Part model, mm, in its own coordinate system. Face numbers are marked on the shaded views. Round coordinates to 2 decimals unless told otherwise and drop trailing zeros. Write each loop counter-clockwise with the first axis right and the second up, starting at its lowest first coordinate (ties: lowest second). Pieces come first, ordered by that corner, then holes. Notation, with made-up numbers: (46, 47.5) -> (103, 47.5) arc R17 ccw to (103, 69.5) -> close; hole circle Ø4 at (71.5, 13). An arc over 180 degrees is marked (long way). Use CSV: the item, a comma, the result in double quotes. Start each with the question number.
(1) Two-plate mould, pull along Z, no slides. Class the marked faces 1, 2, 3 and 4: released by +Z, released by -Z, zero draft, split by the parting line, or undercut.
(2) Saw through at C-C (z = 0.5). Give the cut face in (x, y).
(3) Saw through at A-A (y = 0.9). Give the cut face in (x, z), plus the area to 3 significant figures.
(4) Drop a flat-ended pin along its axis: pin 1 (1.5 mm diameter, centred on x = 0.5, z = 0.5, fed in from -Y). Give the stop position or say it passes through.
(5) Probe line 1 (Z direction, x = -0.75, y = 1.75); line 2 (X direction, y = 1.8, z = 2); line 3 (Y direction, x = -1, z = 0). List the from-to ranges inside material, lowest first. Write a range as [from, to].
(6) Saw through at B-B (x = 1). Give the cut face in (y, z), plus the area to 3 significant figures.
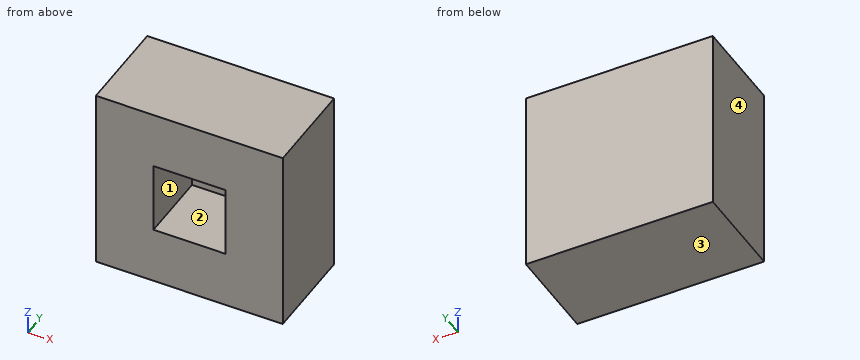
```python
from build123d import *

# Parameters (mm, degrees)
SKETCH1_W           = 7.8
SKETCH1_H           = 7.8
BOSS_EXTRUDE1_DEPTH = 3
SKETCH3_W           = 7.8
SKETCH3_H           = 7.8
BOSS_EXTRUDE2_DEPTH = 1
CUT_EXTRUDE1_DEPTH  = 3


with BuildPart() as part:
    # Sketch1 → Boss-Extrude1 (new body)
    with BuildSketch(Plane(origin=(0, 0, 0), x_dir=(1, 0, 0), z_dir=(0, 1, 0))):
        with Locations((0.315714286, -0.742857143)):
            Rectangle(SKETCH1_W, SKETCH1_H)
    extrude(amount=BOSS_EXTRUDE1_DEPTH)

    # Sketch3 → Boss-Extrude2 (add)
    with BuildSketch(Plane(origin=(0, 3, 0), x_dir=(1, 0, 0), z_dir=(0, 1, 0))):
        with Locations((0.315714286, -0.742857143)):
            Rectangle(SKETCH3_W, SKETCH3_H)
    extrude(amount=BOSS_EXTRUDE2_DEPTH)

    # Sketch4 → Cut-Extrude1 (cut)
    with BuildSketch(Plane.XZ):
        Polygon((0.319353372, 2.24216051), (1.818656739, 2.24216051), (1.818656739, -0.756446224), (-1.179949996, -0.756446224), (-1.179949996, 2.24216051), align=None)
    extrude(amount=-CUT_EXTRUDE1_DEPTH, mode=Mode.SUBTRACT)


solid = part.part
```
Answers:
1,face 1,"undercut"
1,face 2,"undercut"
1,face 3,"released by -Z"
1,face 4,"zero draft"
2,outline,"(-3.58, 0) -> (-1.18, 0) -> (-1.18, 3) -> (1.82, 3) -> (1.82, 0) -> (4.22, 0) -> (4.22, 4) -> (-3.58, 4) -> close"
3,outline,"(-3.58, -3.16) -> (4.22, -3.16) -> (4.22, 4.64) -> (-3.58, 4.64) -> close; hole (-1.18, -0.76) -> (1.82, -0.76) -> (1.82, 2.24) -> (-1.18, 2.24) -> close"
3,area,"51.8 mm²"
4,pin 1,"stops at y = 3"
5,line 1,"z = [-3.16, -0.76], [2.24, 4.64]"
5,line 2,"x = [-3.58, -1.18], [1.82, 4.22]"
5,line 3,"y = [3, 4]"
6,outline,"(0, -3.16) -> (4, -3.16) -> (4, 4.64) -> (0, 4.64) -> (0, 2.24) -> (3, 2.24) -> (3, -0.76) -> (0, -0.76) -> close"
6,area,"22.2 mm²"
